The listing builds one solid part. Answer for the finished solid, in the listing's coordinates (mm). Give positions to 0.01 mm unless a question says otherwise; leave off trailing zeros. Order: outer loops, then holes, each group sorted by start corner. A loop starts at its lowest first (then second) coordinate and runs counter-clockwise, first axis right, second up. Notation, with made-up numbers: (57, -8) -> (115, -8) arc R26 cw to (115, 17) -> close; hole circle Ø9 at (57, 78.5). An arc over 180 degrees is marked (long way). Write item = value, one per line. Start each with the question number.
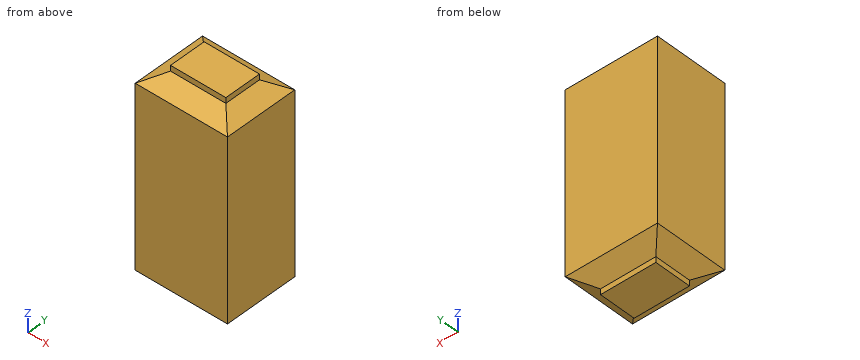
```python
from build123d import *

# Parameters (mm, degrees)
SKETCH1_W           = 50
SKETCH1_H           = 40
BOSS_EXTRUDE1_DEPTH = 115


with BuildPart() as part:
    # Sketch1 → Boss-Extrude1 (new body)
    with BuildSketch(Plane.XY):
        Rectangle(SKETCH1_W, SKETCH1_H)
    extrude(amount=-BOSS_EXTRUDE1_DEPTH)

    # Cut-Sweep1: sweep along a path in Sketch2
    with BuildLine(Plane.XY) as cut_sweep1_path:
        Line((-15, -10), (15, -10))
        Line((15, -10), (15, 10))
        Line((15, 10), (-15, 10))
        Line((-15, 10), (-15, -10))
    # Sketch3 → Cut-Sweep1 (sweep, cut)
    with BuildSketch(Plane(origin=(15, 10, 0), x_dir=(0, 0, -1), z_dir=(1, 0, 0))):
        Polygon((8.773502692, 10), (0, 10), (0, 0), (3, 0), align=None)
    cut_sweep1 = sweep(path=cut_sweep1_path.line, transition=Transition.RIGHT, mode=Mode.SUBTRACT)

    # Mirror1: Cut-Sweep1 across plane
    add(cut_sweep1.mirror(Plane.XY.offset(-57.5)), mode=Mode.SUBTRACT)


solid = part.part
```
Item 1: Flat-ended cylindrical pins translate along their axes: pin 1 (0.9 mm diameter, centred on y = -4, z = -113, fed in from +X); pin 2 (1.5 mm diameter, centred on y = -1, z = -2, fed in from -X); pin 3 (2.5 mm diameter, centred on x = -1, z = -113.5, fed in from +Y). Find the tip coordinate at first contact, or state that the pin passes through.
Item 2: A cutting plane is placed at A-A, the plane y = -1. Write down the section's boundary in (x, z).
Item 3: Consider L1, parallel to Z at x = 21.5, y = -1; L2, parallel to X at y = -6, z = -108; L3, parallel to Z at x = 15.5, y = 8.5. Determine where each line is inside the solid, lowest interval first. Write a range as from..to.
Item 4: A cutting plane is placed at B-B, the plane x = 21. Write down the section's boundary in (y, z).
Item 5: A cutting plane is placed at D-D, the plane y = 11.5. Write down the section's boundary in (x, z), plus the area to 3 significant figures.
Item 6: A cutting plane is placed at C-C, the plane x = -2. Write down the section's boundary in (y, z), plus the area to 3 significant figures.
Check values:
q1.pin_1 = 15
q1.pin_2 = -15
q1.pin_3 = 10
q2.outline = (-25, -106.23) -> (-15, -112) -> (-15, -115) -> (15, -115) -> (15, -112) -> (25, -106.23) -> (25, -8.77) -> (15, -3) -> (15, 0) -> (-15, 0) -> (-15, -3) -> (-25, -8.77) -> close
q3.L1 = -108.25..-6.75
q3.L2 = -21.93..21.93
q3.L3 = -111.71..-3.29
q4.outline = (-20, -106.23) -> (-16, -108.54) -> (16, -108.54) -> (20, -106.23) -> (20, -8.77) -> (16, -6.46) -> (-16, -6.46) -> (-20, -8.77) -> close
q5.outline = (-25, -106.23) -> (-16.5, -111.13) -> (16.5, -111.13) -> (25, -106.23) -> (25, -8.77) -> (16.5, -3.87) -> (-16.5, -3.87) -> (-25, -8.77) -> close
q5.area = 5,280 mm^2
q6.outline = (-20, -106.23) -> (-10, -112) -> (-10, -115) -> (10, -115) -> (10, -112) -> (20, -106.23) -> (20, -8.77) -> (10, -3) -> (10, 0) -> (-10, 0) -> (-10, -3) -> (-20, -8.77) -> close
q6.area = 4,360 mm^2
